Can you work these out from the drawing? Everything is in mm from the part's minimum corner. Round coordinates to 2 decimals unless told otherwise and drop trailing zeros. Write each loop counter-clockwise with the first axis right and the second up, starting at its lowest first coordinate (ties: lowest second). Pieces come first, ordered by that corner, then holes. Notation, with made-up numbers: (78, -2.75) -> (116, -2.75) arc R18 ccw to (116, 20.25) -> close; hole circle Ø3 at (18.5, 6.5). An arc over 180 degrees is marked (long way). Answer as CSV lines item,"result".
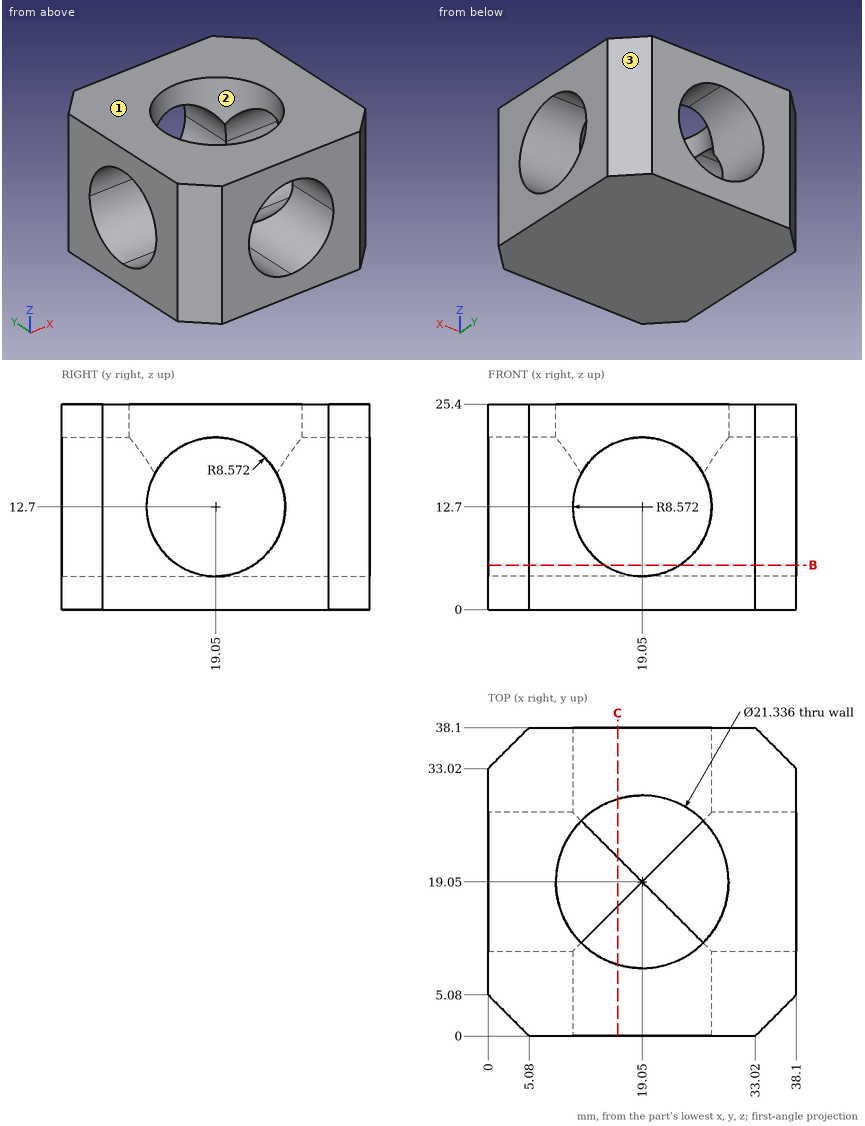
Item 1: If we mould it in two halves opening along X, with no side actions, what happens to the marked faces 1, 2 and 3? For each: pulls with the +X half, pulls with the -X half, needs draft (parallel to the pull), parting line crosses it, or undercut.
Results found:
face 1,"needs draft"
face 2,"undercut"
face 3,"pulls with the +X half"
Item 2: Suppose I cut it at B-B, the plane z = 5.5. List the corners of the cut face in (x, y) for me.
Results found:
outline,"(0, 5.08) -> (5.08, 0) -> (14.4, 0) -> (14.4, 14.4) -> (0, 14.4) -> close; (0, 23.7) -> (14.4, 23.7) -> (14.4, 38.1) -> (5.08, 38.1) -> (0, 33.02) -> close; (23.7, 0) -> (33.02, 0) -> (38.1, 5.08) -> (38.1, 14.4) -> (23.7, 14.4) -> close; (23.7, 23.7) -> (38.1, 23.7) -> (38.1, 33.02) -> (33.02, 38.1) -> (23.7, 38.1) -> close"
Item 3: Suppose I cut it at C-C, the plane x = 16. State how many separate pieces and enclosed holes the cut face has, then the cut area to 3 significant figures.
Results found:
separate pieces,"3"
enclosed holes,"0"
area,"259 mm²"
Item 4: I need wall thicknesses on L1, parallel to X at y = 32.5, z = 12.5; L2, parallel to Y at x = 19.05, z = 23.75; L3, parallel to X at y = 14.5, z = 21.5. Which ranges of each line are inside material? Lowest first, please.
Results found:
L1,"x = 0 to 10.48, 27.62 to 38.1"
L2,"y = 0 to 8.38, 29.72 to 38.1"
L3,"x = 0 to 9.4, 28.7 to 38.1"
